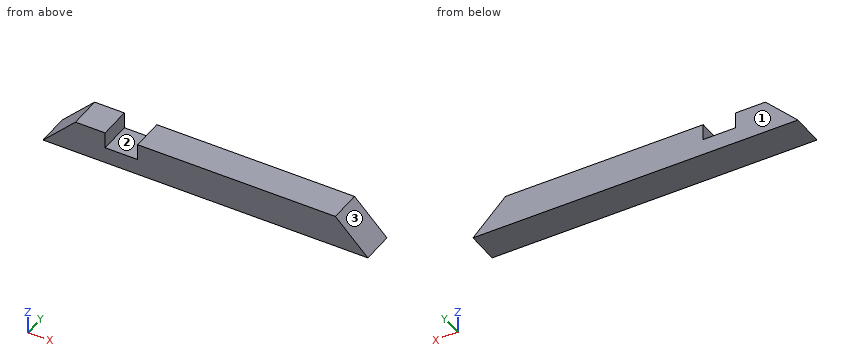
from build123d import *

# Parameters (mm, degrees)
F0_W     = 254
F0_H     = 25.4
F1_DEPTH = 25.4
F2_SIZE2 = 25.39999
F2_SIZE  = 25.39999
F3_SIZE2 = 25.39999
F3_SIZE  = 25.39999
F4_W     = 25.4
F4_H     = 25.4
F5_DEPTH = 12.7


# Not quite as in the source:
# - a fillet or chamfer is up to 0.001 mm smaller than in the source, because OpenCascade refuses the exact size


with BuildPart() as f1:
    # F0 (on Front) → F1 (new body)
    with BuildSketch(Plane.XZ):
        with Locations((52.2324490321, -35.310111469)):
            Rectangle(F0_W, F0_H)
    extrude(amount=-F1_DEPTH)

    # F2 (size 25.4 and 25.4 in the source; OpenCascade refuses exactly that, so slightly less here)
    f2_edges = [f1.edges().sort_by_distance(p)[0] for p in [
        (179.232449, 12.7, -22.610111),
    ]]
    chamfer(f2_edges, length=F2_SIZE, length2=F2_SIZE2)

    # F3 (size 25.4 and 25.4 in the source; OpenCascade refuses exactly that, so slightly less here)
    f3_edges = [f1.edges().sort_by_distance(p)[0] for p in [
        (-74.767551, 12.7, -22.610111),
    ]]
    chamfer(f3_edges, length=F3_SIZE, length2=F3_SIZE2)

    # F4 (on face) → F5 (cut)
    with BuildSketch(Plane.XY.offset(-22.610111469)):
        with Locations((-13.4418782175, 12.7)):
            Rectangle(F4_W, F4_H)
    extrude(amount=-F5_DEPTH, mode=Mode.SUBTRACT)


solid = f1.part
The model under review builds one solid part; all positions refer to its coordinate system, in mm. Face numbers are marked on the shaded views. Give positions to 0.01 mm unless a question says otherwise; leave off trailing zeros. Loops run counter-clockwise (first coordinate to the right, second up) from the corner with the lowest first, then second, coordinate; pieces in that order, holes last. Notation, with made-up numbers: (87.25, -10.75) -> (126.25, -10.75) arc R12 cw to (126.25, -3.75) -> close; hole circle Ø9 at (1, 74). An arc over 180 degrees is marked (long way). Write each question's results on one line, items separated by ' | '.
1) Take a section at A-A, the plane z = -27.75. Give the boundary of the cut face in (x, y).
Conclusion:
outline: (-54.51, 0) -> (-26.14, 0) -> (-26.14, 25.4) -> (-54.51, 25.4) -> close; (-0.74, 0) -> (158.97, 0) -> (158.97, 25.4) -> (-0.74, 25.4) -> close
2) Draft analysis for pull direction X (two halves, no side actions). For the marked faces 1, 2 and 3, state which applies: pulls with the +X half, pulls with the -X half, needs draft (parallel to the pull), parting line crosses it, or undercut.
Conclusion:
face 1: needs draft | face 2: undercut | face 3: pulls with the +X half
3) For line 1 along Z through (x, y) = (-24.5, 7.5); line 2 along X through (y, z) = (10.25, -27.25); line 3 along X through (y, z) = (11.75, -28), list the stretches that pass through material, from the lowest coordinate up. Write a range as from..to.
Conclusion:
line 1: z = -48.01..-35.31 | line 2: x = -54.01..-26.14, -0.74..158.47 | line 3: x = -54.76..-26.14, -0.74..159.22
4) Take a section at D-D, the plane z = -40.25. Give the boundary of the cut face in (x, y).
Conclusion:
outline: (-67.01, 0) -> (171.47, 0) -> (171.47, 25.4) -> (-67.01, 25.4) -> close
5) Insertion check: pin 1 Ø5 at (y, z) = (3.5, -33) entering from -X; pin 2 Ø14 at (y, z) = (6.5, -28) entering from +X; pin 3 Ø10 at (y, z) = (19.5, -31) entering from -X. Each pin has a flat end and moves straight along its axis. Give the tip position at first contact, or say it passes through.
Conclusion:
pin 1: stops at x = -62.26 | pin 2: stops at x = 166.22 | pin 3: stops at x = -62.76
